```python
from build123d import *

# Parameters (mm, degrees)
BOSS_EXTRUDE1_DEPTH = 50


with BuildPart() as part:
    # Sketch4 → Boss-Extrude1 (new body)
    with BuildSketch(Plane.XY):
        with BuildLine():
            ThreePointArc((4.968986099, 0.120803098), (5.101132242, 0.098182628), (5.233497909, 0.076884301))
            ThreePointArc((5.233497909, 0.076884301), (6.972697635, 2.203383358), (7.139946857, 4.945433981))
            ThreePointArc((7.139946857, 4.945433981), (8.434999235, 4.888713692), (9.730051613, 4.945433981))
            ThreePointArc((9.730051613, 4.945433981), (9.897300835, 2.203383358), (11.636500561, 0.076884301))
            ThreePointArc((11.636500561, 0.076884301), (11.768866228, 0.098182628), (11.901012371, 0.120803098))
            ThreePointArc((11.901012371, 0.120803098), (12.032925783, 0.144743452), (12.16459328, 0.170001296))
            ThreePointArc((12.16459328, 0.170001296), (13.0716304, 2.764324962), (12.289539875, 5.399010148))
            ThreePointArc((12.289539875, 5.399010148), (13.501291083, 5.782037637), (14.675751687, 6.26752022))
            ThreePointArc((14.675751687, 6.26752022), (15.77017858, 3.746516175), (18.132608433, 2.342181169))
            ThreePointArc((18.132608433, 2.342181169), (18.366147116, 2.473919706), (18.597005377, 2.61030087))
            ThreePointArc((18.597005377, 2.61030087), (18.562422416, 5.35722969), (16.927986588, 7.56526806))
            ThreePointArc((16.927986588, 7.56526806), (17.946753802, 8.346079322), (18.894100505, 9.212155005))
            ThreePointArc((18.894100505, 9.212155005), (20.784759544, 7.217502149), (23.485028304, 6.705857505))
            ThreePointArc((23.485028304, 6.705857505), (23.659425648, 6.909526169), (23.829716347, 7.116640718))
            ThreePointArc((23.829716347, 7.116640718), (22.857714006, 9.686081391), (20.566653119, 11.201948778))
            ThreePointArc((20.566653119, 11.201948778), (21.256927973, 12.284110268), (21.850927349, 13.421966851))
            ThreePointArc((21.850927349, 13.421966851), (24.309777153, 12.194249757), (27.022192556, 12.637007368))
            ThreePointArc((27.022192556, 12.637007368), (27.116413667, 12.888040714), (27.205597232, 13.140907576))
            ThreePointArc((27.205597232, 13.140907576), (25.413413337, 15.222947636), (22.742063147, 15.863808061))
            ThreePointArc((22.742063147, 15.863808061), (23.020588306, 17.116795131), (23.189595265, 18.389190318))
            ThreePointArc((23.189595265, 18.389190318), (25.920062258, 18.076489787), (28.317466974, 19.420246552))
            ThreePointArc((28.317466974, 19.420246552), (28.320147397, 19.688366252), (28.317466974, 19.956485953))
            ThreePointArc((28.317466974, 19.956485953), (25.921265354, 21.30000064), (23.191830118, 20.988556878))
            ThreePointArc((23.191830118, 20.988556878), (23.025011337, 22.261240797), (22.748641145, 23.514704949))
            ThreePointArc((22.748641145, 23.514704949), (25.42139071, 24.154737279), (27.21462235, 26.2374163))
            ThreePointArc((27.21462235, 26.2374163), (27.125438785, 26.490283162), (27.031217673, 26.741316508))
            ThreePointArc((27.031217673, 26.741316508), (24.320015606, 27.184258124), (21.861705497, 25.958074888))
            ThreePointArc((21.861705497, 25.958074888), (21.269663582, 27.096951192), (20.581250564, 28.180298033))
            ThreePointArc((20.581250564, 28.180298033), (22.873909658, 29.695865881), (23.84667802, 32.26626533))
            ThreePointArc((23.84667802, 32.26626533), (23.676387321, 32.473379879), (23.501989977, 32.677048544))
            ThreePointArc((23.501989977, 32.677048544), (20.802798446, 32.165991792), (18.912121943, 30.172964878))
            ThreePointArc((18.912121943, 30.172964878), (17.966265888, 31.040668276), (16.948842813, 31.82323019))
            ThreePointArc((16.948842813, 31.82323019), (18.584882913, 34.031533704), (18.619857777, 36.779625474))
            ThreePointArc((18.619857777, 36.779625474), (18.388999516, 36.916006638), (18.155460833, 37.047745174))
            ThreePointArc((18.155460833, 37.047745174), (15.793842173, 35.644331042), (14.698842765, 33.124848909))
            ThreePointArc((14.698842765, 33.124848909), (13.51325677, 33.616721566), (12.289539875, 34.004110035))
            ThreePointArc((12.289539875, 34.004110035), (13.0716304, 36.638795221), (12.16459328, 39.233118887))
            ThreePointArc((12.16459328, 39.233118887), (11.901012371, 39.282317085), (11.636500561, 39.326235881))
            ThreePointArc((11.636500561, 39.326235881), (9.897300835, 37.199736825), (9.730051613, 34.457686202))
            ThreePointArc((9.730051613, 34.457686202), (8.447734845, 34.514401016), (7.16532245, 34.459891274))
            ThreePointArc((7.16532245, 34.459891274), (6.99913174, 37.203176215), (5.259484699, 39.330818054))
            ThreePointArc((5.259484699, 39.330818054), (4.994972889, 39.286899257), (4.73139198, 39.237701059))
            ThreePointArc((4.73139198, 39.237701059), (3.824384344, 36.644604248), (4.605058031, 34.010716908))
            ThreePointArc((4.605058031, 34.010716908), (3.380676818, 33.625433236), (2.194246783, 33.135599963))
            ThreePointArc((2.194246783, 33.135599963), (1.09981989, 35.656604008), (-1.262609963, 37.060939014))
            ThreePointArc((-1.262609963, 37.060939014), (-1.496148646, 36.929200477), (-1.727006907, 36.792819313))
            ThreePointArc((-1.727006907, 36.792819313), (-1.692423946, 34.045890493), (-0.057988118, 31.837852122))
            ThreePointArc((-0.057988118, 31.837852122), (-1.076755332, 31.05704086), (-2.024102035, 30.190965178))
            ThreePointArc((-2.024102035, 30.190965178), (-3.914761075, 32.185618033), (-6.615029835, 32.697262678))
            ThreePointArc((-6.615029835, 32.697262678), (-6.789427179, 32.493594014), (-6.959717877, 32.286479465))
            ThreePointArc((-6.959717877, 32.286479465), (-5.987715536, 29.717038792), (-3.696654649, 28.201171405))
            ThreePointArc((-3.696654649, 28.201171405), (-4.386929503, 27.119009915), (-4.980928879, 25.981153332))
            ThreePointArc((-4.980928879, 25.981153332), (-7.439778683, 27.208870426), (-10.152194086, 26.766112815))
            ThreePointArc((-10.152194086, 26.766112815), (-10.246415197, 26.515079469), (-10.335598762, 26.262212607))
            ThreePointArc((-10.335598762, 26.262212607), (-8.543414868, 24.180172547), (-5.872064677, 23.539312122))
            ThreePointArc((-5.872064677, 23.539312122), (-6.150589836, 22.286325051), (-6.319596795, 21.013929865))
            ThreePointArc((-6.319596795, 21.013929865), (-9.050063788, 21.326630396), (-11.447468504, 19.982873631))
            ThreePointArc((-11.447468504, 19.982873631), (-11.450148927, 19.714753931), (-11.447468504, 19.44663423))
            ThreePointArc((-11.447468504, 19.44663423), (-9.051266884, 18.103119543), (-6.321831648, 18.414563305))
            ThreePointArc((-6.321831648, 18.414563305), (-6.155012867, 17.141879386), (-5.878642675, 15.888415234))
            ThreePointArc((-5.878642675, 15.888415234), (-8.55139224, 15.248382904), (-10.34462388, 13.165703883))
            ThreePointArc((-10.34462388, 13.165703883), (-10.255440315, 12.91283702), (-10.161219203, 12.661803675))
            ThreePointArc((-10.161219203, 12.661803675), (-7.450017136, 12.218862059), (-4.991707027, 13.445045295))
            ThreePointArc((-4.991707027, 13.445045295), (-4.399665112, 12.306168991), (-3.711252094, 11.222822149))
            ThreePointArc((-3.711252094, 11.222822149), (-6.003911188, 9.707254302), (-6.97667955, 7.136854852))
            ThreePointArc((-6.97667955, 7.136854852), (-6.806388851, 6.929740303), (-6.631991507, 6.726071639))
            ThreePointArc((-6.631991507, 6.726071639), (-3.932799977, 7.23712839), (-2.042123473, 9.230155305))
            ThreePointArc((-2.042123473, 9.230155305), (-1.096267418, 8.362451907), (-0.078844343, 7.579889993))
            ThreePointArc((-0.078844343, 7.579889993), (-1.714884443, 5.371586479), (-1.749859307, 2.623494709))
            ThreePointArc((-1.749859307, 2.623494709), (-1.519001046, 2.487113545), (-1.285462363, 2.355375008))
            ThreePointArc((-1.285462363, 2.355375008), (1.076156297, 3.758789141), (2.171155705, 6.278271274))
            ThreePointArc((2.171155705, 6.278271274), (3.3567417, 5.786398617), (4.580458595, 5.399010148))
            ThreePointArc((4.580458595, 5.399010148), (3.79836807, 2.764324962), (4.705405189, 0.170001296))
            ThreePointArc((4.705405189, 0.170001296), (4.837072687, 0.144743452), (4.968986099, 0.120803098))
        make_face()
    extrude(amount=BOSS_EXTRUDE1_DEPTH)


solid = part.part
```
Verification items for the finished model (mm, model axes). Coordinates: 2 decimals unless noted, no trailing zeros. Write each loop counter-clockwise with the first axis right and the second up, starting at its lowest first coordinate (ties: lowest second). Pieces come first, ordered by that corner, then holes. Notation, with made-up numbers: M 21.5,61 L 40.5,61 A18 ccw 40.5,80 Z; hole C -16.75,22.5 d4. An arc over 180 degrees is marked long. Answer as a JSON object with one key per item and string values. Group by question number.
(1) Material ranges on line 1 (Y direction, x = 24.5, z = 16); line 2 (Y direction, x = 26, z = 24.5); line 3 (X direction, y = 8.5, z = 19.5), recorded low to high.
(2) Cross-section at B-B, the plane x = 11. Record the cut outline in (y, z).
(3) Cross-section at C-C, the plane y = 25. Record the cut outline in (x, z), and give its area (3 significant figures).
(4) Gauge pin test, flat end, axial feed: pin 1 (5 mm diameter, centred on y = 14.5, z = 28.5, fed in from -X). Record the tip position at first contact, or that the pin passes through.
(5) Cross-section at A-A, the plane y = 31. Record the cut outline in (x, z), and give its area (3 significant figures).
(6) Release check for a two-part mould opening along X. For faces 1 (the face through (17.93, 8.33, 24.65)), 2 (the face through (8, 20, 50)), 3 (the face through (3.398, 33.632, 24.65)) record: +X half, -X half, draft (parallel to the pull), parting line (faces both ways), or undercut.
Reply:
{
 "1": {"line 1": "12.17 to 15.65, 18.02 to 21.36, 23.73 to 27.21", "line 2": "12.26 to 14.8, 18.09 to 21.28, 24.57 to 27.12", "line 3": "-6.69 to -2.48, -1.26 to 18.13, 19.32 to 23.54"},
 "2": {"outline": "M 0.57,0 L 38.83,0 L 38.83,50 L 0.57,50 Z"},
 "3": {"outline": "M -9.53,0 L 26.43,0 L 26.43,50 L -9.53,50 Z", "area": "1,800 mm²"},
 "4": {"pin 1": "x = -10.34"},
 "5": {"outline": "M -6.7,0 L -2.52,0 L -2.52,50 L -6.7,50 Z; M -1.14,0 L 18.01,0 L 18.01,50 L -1.14,50 Z; M 19.43,0 L 23.6,0 L 23.6,50 L 19.43,50 Z", "area": "1,380 mm²"},
 "6": {"face 1": "undercut", "face 2": "draft", "face 3": "undercut"}
}
